The listing builds one solid part. Answer for the finished solid, in the listing's coordinates (mm). A direction names the side the tool comes from. Round coordinates to 2 decimals unless told otherwise and drop trailing zeros. Write each loop counter-clockwise with the first axis right and the second up, starting at its lowest first coordinate (ties: lowest second). Pieces come first, ordered by that corner, then holes. Notation, with made-up numbers: (88, 31.5) - (125, 31.5) arc R23 ccw to (125, 60.5) - close; hole circle Ø5 at (-40, -20.5). An arc over 180 degrees is marked (long way). Use a Markdown table: item, result. Add a question column.
1) A tool of negligible diameter and unlimited length cuts with its end or side. For faces 1 (the flat face through (49, 79, 13.296)), 2 (the flat face through (71, 51.845, 73)), 3 (the flat face through (37, 62, 98.296)), 4 (the flat face through (34, 1.845, 38)), 5 (the cylindrical face through (33.29, 83.39, 93.37)), from which of +Z, -Z, +X, -X, +Y, -Y can it reach the whole face along a straight path? Write none if from no direction.
2) Determine the mould class of faces 6 (the flat face through (73, 27, 48.296)), 7 (the flat face through (49, 74.345, 18)), 8 (the cylindrical face through (51.351, 48.838, 72.946)) for opening direction Y: +Y half, -Y half, draft (parallel to the pull), parting line (faces both ways), or undercut.
3) A cutting plane is placed at C-C (y = 79.5). Give the vertices of the cut face in (x, z).
4) A cutting plane is placed at B-B (z = 53.5). Give the vertices of the cut face in (x, y), then the cut area to 3 significant figures.
5) A cutting plane is placed at D-D (y = 30). Give the vertices of the cut face in (x, z), then the cut area to 3 significant figures.
6) Find the intervals of material crossed by probe 1 along Y at (x, z) = (86.5, 17); probe 2 along Z at (x, y) = (83, 81); probe 3 along Z at (x, y) = (16, 42), in increasing order. Write a range as from..to.
7) A cutting plane is placed at A-A (x = 68.5). Give the vertices of the cut face in (y, z).
8) Each of these flat-tipped pins is pushed along its axis until it touches: P1, Ø1, axis at y = 49.5, z = 85.5, coming from the +X side; P2, Ø8, axis at x = 31.5, y = 77.5, coming from the +Z side; P3, Ø12.5, axis at y = 32.5, z = 71, coming from the +X side. Where does it stop, or does it pass through?
```python
from build123d import *

# Parameters (mm, degrees)
F1_DEPTH  = 50
F2_DEPTH  = 50
F3_R      = 12.5
F4_DEPTH  = 10
F5_DEPTH  = 10
F6_W      = 10
F6_H      = 10
F7_DEPTH  = 100
F8_DEPTH  = 100
F9_DEPTH  = 100
F11_ANGLE = 90


with BuildPart() as f1:
    # F0 (on Right) → F1 (new body)
    with BuildSketch(Plane.YZ):
        with BuildLine():
            Line((66.8447806998, -31.704402437), (66.8447806998, 68.295597563))
            Line((66.8447806998, 68.295597563), (-33.1552193002, 68.295597563))
            Line((-33.1552193002, 68.295597563), (-33.1552193002, 33.295597563))
            Line((-33.1552193002, 33.295597563), (-18.1553634487, 18.2957411159))
            Line((-18.1553634487, 18.2957411159), (6.8449245505, 18.2957411159))
            ThreePointArc((6.8449245505, 18.2957411159), (13.9159923623, 15.3668089278), (16.8449245505, 8.2957411159))
            Line((16.8449245505, 8.2957411159), (16.8449245505, -16.7045462877))
            Line((16.8449245505, -16.7045462877), (31.8447806998, -31.704402437))
            Line((31.8447806998, -31.704402437), (66.8447806998, -31.704402437))
        make_face()
    extrude(amount=F1_DEPTH)

    # F1_face (on face) + F0 (on Right) → F2 (join)
    with BuildSketch(Plane(origin=(0, 26.0207710076, 27.4715879225), x_dir=(0, 1, 0), z_dir=(-1, 0, 0))):
        with BuildLine():
            Line((40.8240096922, -40.8240096405), (40.8240096922, 59.1759903595))
            Line((40.8240096922, 59.1759903595), (5.8240096922, 59.1759903595))
            Line((5.8240096922, 59.1759903595), (-9.1758464571, 44.1761342102))
            Line((-9.1758464571, 44.1761342102), (-9.1758464571, 19.1758468066))
            ThreePointArc((-9.1758464571, 19.1758468066), (-12.1047786452, 12.1047789947), (-19.1758464571, 9.1758468066))
            Line((-19.1758464571, 9.1758468066), (-44.1761344563, 9.1758468066))
            Line((-44.1761344563, 9.1758468066), (-59.1759903078, -5.8240096405))
            Line((-59.1759903078, -5.8240096405), (-59.1759903078, -40.8240096405))
            Line((-59.1759903078, -40.8240096405), (40.8240096922, -40.8240096405))
        make_face()
    with BuildSketch(Plane.YZ):
        with BuildLine():
            Line((66.8447806998, -31.704402437), (66.8447806998, 68.295597563))
            Line((66.8447806998, 68.295597563), (-33.1552193002, 68.295597563))
            Line((-33.1552193002, 68.295597563), (-33.1552193002, 33.295597563))
            Line((-33.1552193002, 33.295597563), (-18.1553634487, 18.2957411159))
            Line((-18.1553634487, 18.2957411159), (6.8449245505, 18.2957411159))
            ThreePointArc((6.8449245505, 18.2957411159), (13.9159923623, 15.3668089278), (16.8449245505, 8.2957411159))
            Line((16.8449245505, 8.2957411159), (16.8449245505, -16.7045462877))
            Line((16.8449245505, -16.7045462877), (31.8447806998, -31.704402437))
            Line((31.8447806998, -31.704402437), (66.8447806998, -31.704402437))
        make_face()
        with BuildLine():
            Line((-18.1553634487, 18.2957411159), (-33.1552193002, 33.295597563))
            Line((-33.1552193002, 33.295597563), (-33.1552193002, -21.704402437))
            ThreePointArc((-33.1552193002, -21.704402437), (-30.2262871121, -28.7754702488), (-23.1552193002, -31.704402437))
            Line((-23.1552193002, -31.704402437), (31.8447806998, -31.704402437))
            Line((31.8447806998, -31.704402437), (16.8449245505, -16.7045462877))
            Line((16.8449245505, -16.7045462877), (16.8449245505, 8.2957411159))
            ThreePointArc((16.8449245505, 8.2957411159), (13.9159923623, 15.3668089278), (6.8449245505, 18.2957411159))
            Line((6.8449245505, 18.2957411159), (-18.1553634487, 18.2957411159))
        make_face()
    extrude(amount=F2_DEPTH, dir=(-1, 0, 0))

    # F3 (on face) → F4 (join)
    with BuildSketch(Plane.YZ.offset(50)):
        with Locations((36.8447806998, 38.295597563)):
            Circle(F3_R)
    extrude(amount=-F4_DEPTH)

    # F3 (on face) → F5 (cut)
    with BuildSketch(Plane.YZ.offset(50)):
        with Locations((36.8447806998, 38.295597563)):
            Circle(F3_R)
    extrude(amount=-F5_DEPTH, mode=Mode.SUBTRACT)

    # F6 (on face) → F7 (cut)
    with BuildSketch(Plane(origin=(0, 0, -31.704402437), x_dir=(1, 0, 0), z_dir=(0, 0, -1))):
        with Locations((-30, -6.8447806998)):
            Rectangle(F6_W, F6_H)
    extrude(amount=-F7_DEPTH, mode=Mode.SUBTRACT)

    # F6 (on face) → F8 (cut)
    with BuildSketch(Plane(origin=(0, 0, -31.704402437), x_dir=(1, 0, 0), z_dir=(0, 0, -1))):
        with Locations((7.5, -44.3447806998)):
            Rectangle(F6_W, F6_H)
    extrude(amount=-F8_DEPTH, mode=Mode.SUBTRACT)

    # F6 (on face) → F9 (cut)
    with BuildSketch(Plane(origin=(0, 0, -31.704402437), x_dir=(1, 0, 0), z_dir=(0, 0, -1))):
        with Locations((-30, -44.3447806998)):
            Rectangle(F6_W, F6_H)
    extrude(amount=-F9_DEPTH, mode=Mode.SUBTRACT)


with BuildPart() as f1_1:
    # F10: moved
    add(f1.part.moved(Location((25, 60, 0))))


with BuildPart() as f1_2:
    # F11: moved
    add(f1_1.part.rotate(Axis((-25, 76.8447806998, 68.295597563), (0, -1, 0)), F11_ANGLE))


with BuildPart() as f1_3:
    # F12: moved
    add(f1_2.part.moved(Location((25, -25, -70))))


with BuildPart() as f1_4:
    # F13: moved
    add(f1_3.part.moved(Location((-1.5, 0, 0))))


solid = f1_4.part
```
Entries:
| question | item | result |
|---|---|---|
| 1 | face 1 | +X, -X |
| 1 | face 2 | +Z, +X, -Y |
| 1 | face 3 | +Z, +X, -X, +Y, -Y |
| 1 | face 4 | +Z, -Z, +X, -X, -Y |
| 1 | face 5 | +Z |
| 2 | face 6 | draft |
| 2 | face 7 | undercut |
| 2 | face 8 | -Y half |
| 3 | outline | (-1.5, -1.7) - (98.5, -1.7) - (98.5, 13.3) - (-1.5, 13.3) - close; (-1.5, 23.3) - (98.5, 23.3) - (98.5, 50.8) - (-1.5, 50.8) - close; (-1.5, 60.8) - (98.5, 60.8) - (98.5, 98.3) - (38.38, 98.3) - (38.38, 88.3) - (18.62, 88.3) - (18.62, 98.3) - (-1.5, 98.3) - close |
| 4 | outline | (-1.5, 1.84) - (33.5, 1.84) - (48.5, 16.84) - (48.5, 41.84) arc R10 cw to (58.5, 51.84) - (83.5, 51.84) - (98.5, 66.84) - (98.5, 74.34) - (-1.5, 74.34) - close; (-1.5, 84.34) - (98.5, 84.34) - (98.5, 101.84) - (-1.5, 101.84) - close |
| 4 | area | 6,300 mm² |
| 5 | outline | (-1.5, -1.7) - (98.5, -1.7) - (98.5, 48.3) - (48.5, 48.3) - (48.5, 98.3) - (-1.5, 98.3) - close |
| 5 | area | 7,500 mm² |
| 6 | probe 1 | y = 1.84..36.84, 46.84..74.34, 84.34..101.84 |
| 6 | probe 2 | z = -1.7..13.3, 23.3..50.8, 60.8..98.3 |
| 6 | probe 3 | z = -1.7..13.3, 23.3..98.3 |
| 7 | outline | (1.84, -1.7) - (101.84, -1.7) - (101.84, 98.3) - (51.84, 98.3) - (51.84, 48.3) - (1.84, 48.3) - close; hole (36.84, 13.3) - (46.84, 13.3) - (46.84, 23.3) - (36.84, 23.3) - close; hole (74.34, 13.3) - (84.34, 13.3) - (84.34, 23.3) - (74.34, 23.3) - close; hole (74.34, 50.8) - (84.34, 50.8) - (84.34, 60.8) - (74.34, 60.8) - close |
| 8 | P1 | stops at x = 52.71 |
| 8 | P2 | stops at z = 88.3 |
| 8 | P3 | stops at x = 48.5 |
